from build123d import *

# Parameters (mm, degrees)
SKETCH1_W                                = 75
SKETCH1_H                                = 80
BOSS_EXTRUDE1_DEPTH                      = 5
CUT_EXTRUDE1_START                       = -6
CUT_EXTRUDE1_DEPTH                       = 7
MIRROR1_START                            = -6
MIRROR1_AT_THE_SECOND_PLANE_COPY_1_DEPTH = 7
CUT_EXTRUDE2_DEPTH                       = 1
CUT_EXTRUDE2_DEPTH_BACK                  = 6
SKETCH5_R                                = 1.5875
CUT_EXTRUDE3_DEPTH                       = 6


with BuildPart() as part:
    # Sketch1 → Boss-Extrude1 (new body)
    with BuildSketch(Plane(origin=(0, 0, 0), x_dir=(0, 0, -1), z_dir=(1, 0, 0))):
        Rectangle(SKETCH1_W, SKETCH1_H)
    extrude(amount=BOSS_EXTRUDE1_DEPTH)

    # Sketch3 → Cut-Extrude1 (cut)
    with BuildSketch(Plane(origin=(5, 0, 0), x_dir=(0, 0, -1), z_dir=(1, 0, 0)).offset(CUT_EXTRUDE1_START)):
        Polygon((-37.5, 20), (-32.5, 20), (-32.5, 35), (-17.5, 35), (-17.5, 40), (-37.5, 40), align=None)
    cut_extrude1 = extrude(amount=CUT_EXTRUDE1_DEPTH, mode=Mode.SUBTRACT)

    # Mirror1: Cut-Extrude1 across plane
    add(cut_extrude1.mirror(Plane.XY), mode=Mode.SUBTRACT)

    # Mirror1 at the second plane: Cut-Extrude1 across plane
    add(cut_extrude1.mirror(Plane.ZX), mode=Mode.SUBTRACT)

    # Mirror1 at the second plane copy 1 sketc → Mirror1 at the second plane copy 1 (cut)
    with BuildSketch(Plane(origin=(5, 0, 0), x_dir=(0, 0, 1), z_dir=(1, 0, 0)).offset(MIRROR1_START)):
        Polygon((-37.5, 20), (-32.5, 20), (-32.5, 35), (-17.5, 35), (-17.5, 40), (-37.5, 40), align=None)
    extrude(amount=MIRROR1_AT_THE_SECOND_PLANE_COPY_1_DEPTH, mode=Mode.SUBTRACT)

    # Sketch4 → Cut-Extrude2 (cut, two sides)
    with BuildSketch(Plane(origin=(5, 0, 0), x_dir=(0, 0, -1), z_dir=(1, 0, 0))) as cut_extrude2_sk:
        with BuildLine():
            Line((-5.5, -40), (-5.5, 18.4125))
            ThreePointArc((-5.5, 18.4125), (-5.035032015, 19.535032015), (-3.9125, 20))
            Line((-3.9125, 20), (0.9125, 20))
            ThreePointArc((0.9125, 20), (2.035032015, 19.535032015), (2.5, 18.4125))
            Line((2.5, 18.4125), (2.5, -40))
            Line((2.5, -40), (-5.5, -40))
        make_face()
    extrude(amount=CUT_EXTRUDE2_DEPTH, mode=Mode.SUBTRACT)
    extrude(cut_extrude2_sk.sketch, amount=-CUT_EXTRUDE2_DEPTH_BACK, mode=Mode.SUBTRACT)

    # Sketch5 → Cut-Extrude3 (cut, through all)
    with BuildSketch(Plane(origin=(5, 0, 0), x_dir=(0, 0, -1), z_dir=(1, 0, 0))):
        with Locations((-17.5, 35)):
            Circle(SKETCH5_R)
        with Locations((-32.5, 20)):
            Circle(SKETCH5_R)
        with Locations((17.5, 35)):
            Circle(SKETCH5_R)
        with Locations((32.5, 20)):
            Circle(SKETCH5_R)
        with Locations((32.5, -20)):
            Circle(SKETCH5_R)
        with Locations((17.5, -35)):
            Circle(SKETCH5_R)
        with Locations((-17.5, -35)):
            Circle(SKETCH5_R)
        with Locations((-32.5, -20)):
            Circle(SKETCH5_R)
    extrude(amount=-CUT_EXTRUDE3_DEPTH, mode=Mode.SUBTRACT)


solid = part.part
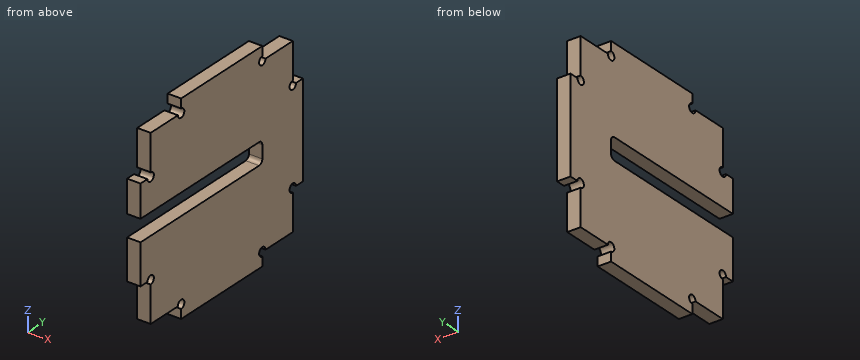
Here's how the part is built. I have some questions about the finished solid (model axes, mm). Coordinates: 2 decimals unless noted, no trailing zeros. Write each loop counter-clockwise with the first axis right and the second up, starting at its lowest first coordinate (ties: lowest second). Pieces come first, ordered by that corner, then holes.
1) If we section it at C-C (z = -20.5): List the corners of the cut face in (x, y) for me, plus the area to 3 significant figures.
Filled in:
outline: (0, -35) - (5, -35) - (5, 35) - (0, 35) - close
area: 350 mm2
2) If I drill on line 1 (Z direction, x = 2.2, y = -2); line 2 (Y direction, x = 1.6, z = 27); line 3 (Y direction, x = 0.6, z = 3.5), over which ranges is the centre line in solid material (lowest first)?
Filled in:
line 1: z = -37.5 to -2.5, 5.5 to 37.5
line 2: y = -35 to 35
line 3: y = 20 to 40
3) If we section it at A-A (y = -1.5): List the corners of the cut face in (x, z) for me.
Filled in:
outline: (0, -37.5) - (5, -37.5) - (5, -2.5) - (0, -2.5) - close; (0, 5.5) - (5, 5.5) - (5, 37.5) - (0, 37.5) - close
4) If we section it at D-D (y = 27): List the corners of the cut face in (x, z) for me.
Filled in:
outline: (0, -32.5) - (5, -32.5) - (5, 32.5) - (0, 32.5) - close
5) I'm going to push flat-ended pins straight in: pin 1 (2.5 mm diameter, centred on x = 3.5, y = 29.5, fed in from -Z); pin 2 (2.5 mm diameter, centred on x = 2.5, y = 38.5, fed in from +Z); pin 3 (2 mm diameter, centred on x = 1, z = -24, fed in from -Y); pin 4 (6 mm diameter, centred on y = -27, z = -28.5, fed in from -X). Where does each tip first touch, or does it pass through?
Filled in:
pin 1: stops at z = -32.5
pin 2: stops at z = 17.5
pin 3: stops at y = -35
pin 4: stops at x = 0
